Drawing for the job (mm, zero at the part's lowest x, y, z). A direction names the side the tool comes from. Coordinates: 2 decimals unless noted, no trailing zeros. Order: outer loops, then holes, each group sorted by start corner. A loop starts at its lowest first (then second) coordinate and runs counter-clockwise, first axis right, second up.
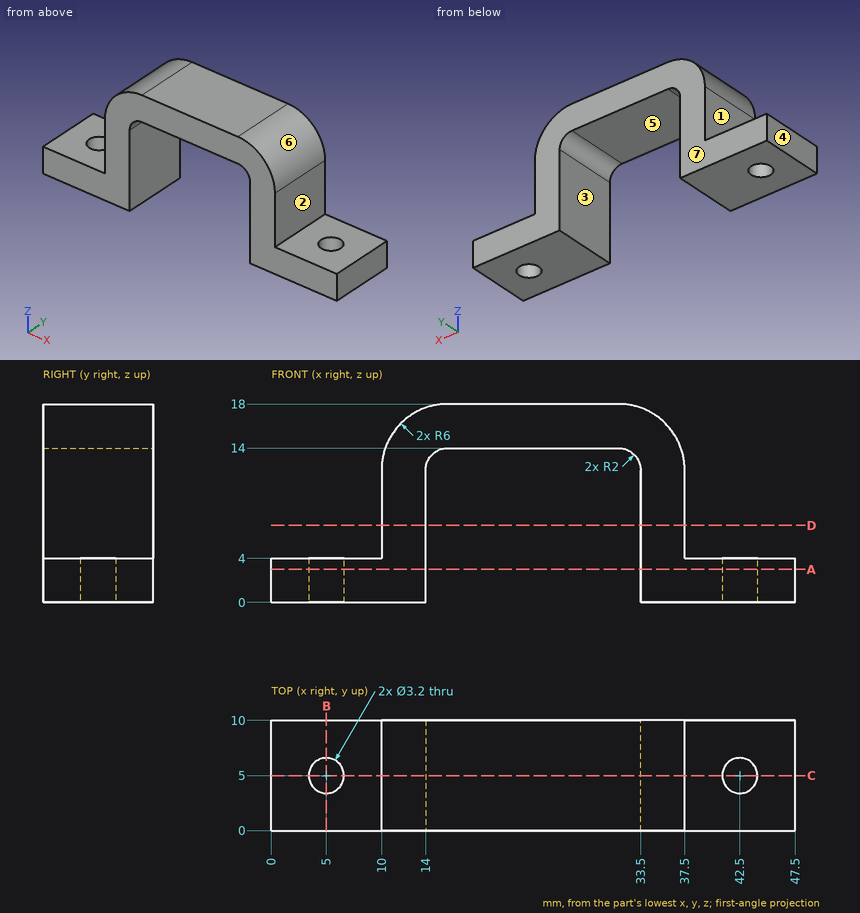
1) Two-plate mould, pull along X, no slides. Class the marked faces 4, 5, 6 and 7: released by +X, released by -X, zero draft, split by the parting line, or undercut.
2) Slice it at A-A (z = 3). List the corners of the cut face in (x, y).
3) Which spindle directions (+Z, -Z, +X, -X, +Y, -Y) get a long thin tool onto all of the face, cutting with end or side? Do the marked faces 1, 2 and 3. Say none if no direction does.
4) Slice it at B-B (x = 5). List the corners of the cut face in (y, z), plus the area to 3 significant figures.
5) Slice it at D-D (z = 7). List the corners of the cut face in (x, y).
6) Drill centre lines: probe 1 along X at (y, z) = (9.75, 11); probe 2 along X at (y, z) = (8.25, 3.25); probe 3 along Y at (x, z) = (42.5, 1.65). Where is each one in solid material? Low to high.
7) Pin check, flat tips, straight feed: P1, Ø2.5, axis at y = 4.5, z = 9.5, coming from the -X side; P2, Ø5, axis at y = 1, z = 10.5, coming from the +X side. Stop position of each tip, or through.
8) Slice it at C-C (y = 5). List the corners of the cut face in (x, z), plus the area to 3 significant figures.
Worked out:
1. face 4: released by -X
1. face 5: undercut
1. face 6: released by +X
1. face 7: zero draft
2. outline: (0, 0) - (14, 0) - (14, 10) - (0, 10) - close; (33.5, 0) - (47.5, 0) - (47.5, 10) - (33.5, 10) - close; hole circle Ø3.2 at (5, 5); hole circle Ø3.2 at (42.5, 5)
3. face 1: +Z, -X, +Y, -Y
3. face 2: +Z, +X, +Y, -Y
3. face 3: -Z, +Y, -Y
4. outline: (0, 0) - (3.4, 0) - (3.4, 4) - (0, 4) - close; (6.6, 0) - (10, 0) - (10, 4) - (6.6, 4) - close
4. area: 27.2 mm2
5. outline: (10, 0) - (14, 0) - (14, 10) - (10, 10) - close; (33.5, 0) - (37.5, 0) - (37.5, 10) - (33.5, 10) - close
6. probe 1: x = 10 to 14, 33.5 to 37.5
6. probe 2: x = 0 to 14, 33.5 to 47.5
6. probe 3: y = 0 to 3.4, 6.6 to 10
7. P1: stops at x = 10
7. P2: stops at x = 37.5
8. outline: (0, 0) - (3.4, 0) - (3.4, 4) - (0, 4) - close; (6.6, 0) - (14, 0) - (14, 12) arc R2 cw to (16, 14) - (31.5, 14) arc R2 cw to (33.5, 12) - (33.5, 0) - (40.9, 0) - (40.9, 4) - (37.5, 4) - (37.5, 12) arc R6 ccw to (31.5, 18) - (16, 18) arc R6 ccw to (10, 12) - (10, 4) - (6.6, 4) - close; (44.1, 0) - (47.5, 0) - (47.5, 4) - (44.1, 4) - close
8. area: 263 mm2
